CAD build for the part. Positions are in the model's coordinates, mm. Give positions to 0.01 mm unless a question says otherwise; leave off trailing zeros. Write each loop counter-clockwise with the first axis right and the second up, starting at its lowest first coordinate (ties: lowest second). Pieces come first, ordered by that corner, then holes. Notation, with made-up numbers: (52.5, 24) -> (94.5, 24) arc R11 ccw to (94.5, 37) -> close; hole circle Ø5 at (60, -19). An arc over 180 degrees is marked (long way). Answer in a Markdown table with one row per item. Add a question column.
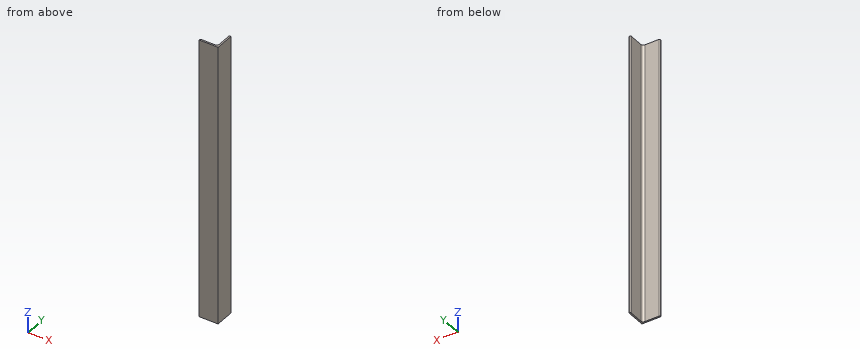
```python
from build123d import *

# Parameters (mm, degrees)
BOSS_EXTRUDE1_DEPTH = 609.6
SKETCH3_W           = 635.2
SKETCH3_H           = 38.1
CUT_EXTRUDE1_DEPTH  = 60
SKETCH4_W           = 20
SKETCH4_H           = 38.1
CUT_EXTRUDE2_DEPTH  = 60


with BuildPart() as part:
    # Sketch2 → Boss-Extrude1 (new, symmetric)
    with BuildSketch(Plane.XY):
        with BuildLine():
            Line((-19.05, -19.05), (19.05, -19.05))
            Line((19.05, -19.05), (19.05, 19.05))
            Line((19.05, 19.05), (17.4625, 19.05))
            ThreePointArc((17.4625, 19.05), (16.339967985, 18.585032015), (15.875, 17.4625))
            Line((15.875, 17.4625), (15.875, -11.0998))
            ThreePointArc((15.875, -11.0998), (14.476376302, -14.476376302), (11.0998, -15.875))
            Line((11.0998, -15.875), (-17.4625, -15.875))
            ThreePointArc((-17.4625, -15.875), (-18.585032015, -16.339967985), (-19.05, -17.4625))
            Line((-19.05, -17.4625), (-19.05, -19.05))
        make_face()
    extrude(amount=BOSS_EXTRUDE1_DEPTH, both=True)

    # Sketch3 → Cut-Extrude1 (cut)
    with BuildSketch(Plane(origin=(19.05, 0, 0), x_dir=(0, 0, -1), z_dir=(1, 0, 0))):
        with Locations((292, 0)):
            Rectangle(SKETCH3_W, SKETCH3_H)
    extrude(amount=-CUT_EXTRUDE1_DEPTH, mode=Mode.SUBTRACT)

    # Sketch4 → Cut-Extrude2 (cut)
    with BuildSketch(Plane(origin=(19.05, 0, 0), x_dir=(0, 0, -1), z_dir=(1, 0, 0))):
        with Locations((-35.6, 0)):
            Rectangle(SKETCH4_W, SKETCH4_H)
    extrude(amount=-CUT_EXTRUDE2_DEPTH, mode=Mode.SUBTRACT)


solid = part.part
```
Item 1: Slice it at C-C, the plane x = -2. List the corners of the cut face in (y, z) (3 decimals), then the cut area to 3 significant figures.
Item 2: Drop flat-ended pins along their axis: pin 1 Ø14.5 at (y, z) = (-3, 467.5) entering from -X (3 decimals); pin 2 Ø2 at (y, z) = (-13, 393) entering from -X. Give the stop position or say it passes through.
Item 3: Slice it at B-B, the plane y = 9. List the corners of the cut face in (x, z) (3 decimals).
Item 4: Probe L1, parallel to X at y = 2, z = 207.5 (3 decimals); L2, parallel to Y at x = -4, z = 267 (3 decimals); L3, parallel to X at y = -12, z = 79. List the from-to ranges inside material, lowest first. Write a range as from..to.
Answer key:
| question | item | result |
|---|---|---|
| 1 | outline | (-19.05, 45.6) -> (-15.875, 45.6) -> (-15.875, 609.6) -> (-19.05, 609.6) -> close |
| 1 | area | 1,790 mm² |
| 2 | pin 1 | stops at x = 15.875 |
| 2 | pin 2 | stops at x = 14.89 |
| 3 | outline | (15.875, 45.6) -> (19.05, 45.6) -> (19.05, 609.6) -> (15.875, 609.6) -> close |
| 4 | L1 | x = 15.875..19.05 |
| 4 | L2 | y = -19.05..-15.875 |
| 4 | L3 | x = 15.79..19.05 |
